Verification items for the finished model (mm, model axes). Give positions to 0.01 mm unless a question says otherwise; leave off trailing zeros. Use CSV: the item, a comma, the result in double quotes. Start each with the question number.
```python
from build123d import *

# Parameters (mm, degrees)
MAIN_BODY_ANGLE    = 180
SKETCH4_R          = 7.488886282
CUT_EXTRUDE3_DEPTH = 314.706


with BuildPart() as part:
    # Sketch1 → main body (revolve)
    with BuildSketch(Plane(origin=(0, 0, 0), x_dir=(1, 0, 0), z_dir=(0, 1, 0))):
        with BuildLine():
            Line((851.304580924, 76.199999981), (1122.351487721, 76.199999981))
            Line((1122.351487721, 76.199999981), (1122.351487721, 1.314116237))
            Line((1122.351487721, 1.314116237), (88.767646843, -9.90077432))
            Line((88.767646843, -9.90077432), (85.047844716, 11.755993253))
            add(Edge.make_bspline(
                [(85.047844716, 11.755993253), (85.832587091, 11.890781898), (87.402836258, 12.159136758), (90.416610596, 12.670807369), (93.537061612, 13.191295846), (97.170324673, 13.792715976), (100.505753233, 14.336151071), (104.017067052, 14.903266848), (107.43124622, 15.44744047), (111.760486229, 16.130713414), (116.925319179, 16.933892159), (122.97234892, 17.858691385), (129.875476741, 18.893918943), (138.513733131, 20.165711278), (148.881759566, 21.656330843), (160.986205499, 23.34879505), (174.826871573, 25.224656034), (192.137141027, 27.502956481), (212.92194706, 30.13846819), (237.187067416, 33.084521174), (264.937120957, 36.294322773), (292.703329319, 39.361555726), (320.48370577, 42.297239812), (348.276817571, 45.109883275), (376.081450756, 47.806042159), (403.896666786, 50.390753056), (431.721669201, 52.867795697), (459.55581535, 55.239882083), (487.398559468, 57.508784018), (515.249450888, 59.675386165), (543.108107682, 61.739743915), (577.940738985, 64.191336351), (612.785340127, 66.468237191), (647.641366116, 68.563465621), (689.481889181, 70.843491315), (724.359891248, 72.534917854), (759.248611408, 73.99264986), (792.5650977, 75.109399967), (814.624980969, 75.693818945), (832.405478938, 76.037890758), (843.204698036, 76.166034998), (848.604594276, 76.201321913), (851.304580924, 76.199999981)],
                knots=[0.087900162, 0.087900162, 0.087900162, 0.087900162, 0.087900162, 0.092039082, 0.096178001, 0.100316921, 0.10445584, 0.10859476, 0.112733679, 0.116872599, 0.121011519, 0.129289358, 0.137567197, 0.145845036, 0.154122875, 0.170678553, 0.18723423, 0.203789907, 0.220345585, 0.253456939, 0.286568294, 0.319679649, 0.352791005, 0.38590236, 0.419013716, 0.45212507, 0.485236425, 0.518347781, 0.551459136, 0.584570491, 0.617681846, 0.650793202, 0.683904557, 0.750127267, 0.783238623, 0.816349978, 0.882572688, 0.915684044, 0.948795399, 0.974397699, 0.98719885, 1, 1, 1, 1, 1], degree=4))
        make_face()
    revolve(axis=Axis((1122.351487721, 0, -1.314116237), (0.9999411386367943, 0, -0.01084985077091772)), revolution_arc=MAIN_BODY_ANGLE)

    # Sketch4 → Cut-Extrude3 (cut)
    with BuildSketch(Plane(origin=(0, 0, 0), x_dir=(0, 0, -1), z_dir=(1, 0, 0))):
        with Locations((-9.90077432, 0)):
            Circle(SKETCH4_R)
    extrude(amount=CUT_EXTRUDE3_DEPTH, mode=Mode.SUBTRACT)


solid = part.part
```
(1) Draft check along Z on faces 1 (the face through (989.535, 76.313, -1.552)), 2 (the face through (87.17, 9.94, 9.7)), 3 (the face through (727, 0, 1)). Enter one of: released by +Z, released by -Z, zero draft, split by the parting line, or undercut.
(2) Thickness scan on line 1 (Y direction, x = 535, z = 18); line 2 (Y direction, x = 1054, z = 58.5); line 3 (Z direction, x = 175, y = 5.5). Record the ranges inside material, lowest first. Write a range as from..to.
(3) Go/stop test with flat-tipped pins: pin 1 (2 mm diameter, centred on y = 4.5, z = 7, fed in from -X); pin 2 (1.5 mm diameter, centred on x = 997.5, y = 13, fed in from +Z); pin 3 (10 mm diameter, centred on x = 916.5, z = 46, fed in from +Y). Record where each tip stops, or that it passes through.
Data:
1,face 1,"split by the parting line"
1,face 2,"undercut"
1,face 3,"zero draft"
2,line 1,"y = 0..64.85"
2,line 2,"y = 0..47.25"
2,line 3,"z = -24.79..4.82, 14.98..42.63"
3,pin 1,"stops at x = 314.71"
3,pin 2,"stops at z = 75.31"
3,pin 3,"stops at y = 65.9"
